Autodesk Inventor part; units mm, degrees
sketch "Sketch19" plane through (0, 0, 0) normal (0, 0, 1) x (1, 0, 0)
  circle A0 centre (0, 0) radius 12.5
  dimension "d130" = 25
extrude "Extrusion17" add sketch "Sketch19" along normal blind 40
sketch "Sketch20" plane through (0, 0, 40) normal (0, 0, 1) x (1, 0, 0)
  circle A0 centre (0, 0) radius 10
  dimension "d133" = 20
fillet "Fillet6" radius 10 1 edges at (-12.5, 0, 0)
extrude "Extrusion18" cut sketch "Sketch20" against normal blind 25
ref_plane "Work Plane3" through (10, 0, 0) normal (1, 0, 0) x (0, 1, 0)
sketch "Sketch21" plane through (10, 0, 0) normal (1, 0, 0) x (0, 1, 0)
  line L0 (0, 0) -> (0, 20)
  circle A0 centre (0, 20) radius 5
  dimension "d138" = 20
  dimension "d139" = 10
extrude "Extrusion19" add sketch "Sketch21" along normal blind 10
mirror "Mirror1" about plane through (0, 0, 0) normal (1, 0, 0) of "Extrusion19"
sketch "Sketch22" plane through (-20, 0, 20) normal (-1, 0, 0) x (0, 0, 1)
  circle A0 centre (0, 0) radius 2.5
  point P0 (-20, 0)
  dimension "d142" = 5
extrude "Extrusion20" cut sketch "Sketch22" against normal blind 3
sketch "Sketch26" plane through (0, 0, 0) normal (1, 0, 0) x (0, 1, 0)
  line L0 (-10, 40) -> (10, 40)
  line L1 (12.5, 40) -> (-12.5, 40)
  line L2 (10, 40) -> (12.5, 40)
  line L3 (17.5, 60) -> (12.5, 40)
  line L4 (17.5, 60) -> (17.5, 62.5)
  line L5 (17.5, 62.5) -> (15, 62.5)
  line L6 (15, 62.5) -> (15, 60)
  line L7 (10, 40) -> (15, 60)
  line L8 (0, -10.5) -> (0, 63)
  point P0 (0, 0)
  dimension "d147" = 2.5
  dimension "d148" = 2.5
revolve "Revolution1" add sketch "Sketch26" angle 360 about axis through (0, 0, -10) along (0, 0, 1)
sketch "Sketch27" plane through (0, 0, 0) normal (1, 0, 0) x (0, 1, 0)
  line L0 (12.5, 40) -> (13.7856, 41.5321)
  line L1 (12.5, 40) -> (14.5, 40) construction
  line L2 (13.7856, 41.5321) -> (17.5, 60)
  line L3 (12.5, 40) -> (-12.5, 40)
  line L4 (12.5, 40) -> (11.5, 40)
  line L5 (-17.5, 60) -> (17.5, 60)
  line L6 (17.5, 60) -> (16.5, 60)
  line L7 (16.5, 60) -> (11.5, 40)
  point P0 (0, 0)
  dimension "d150" = 2
  dimension "d151" = 50
  dimension "d152" = 1
  dimension "d153" = 1
extrude "Extrusion21" add sketch "Sketch27" along normal mid plane 2
pattern_circular "Circular Pattern2" count 8 over 360 about axis through (0, 0, -10) along (0, 0, 1) of "Extrusion21"
properties part number "Waterkanon" material "S235"
The listing builds one solid part. Answer for the finished solid, in the listing's coordinates (mm). A direction names the side the tool comes from. Coordinates: 2 decimals unless noted, no trailing zeros. Loops run counter-clockwise (first coordinate to the right, second up) from the corner with the lowest first, then second, coordinate; pieces in that order, holes last. Notation, with made-up numbers: (5.25, 63.5) -> (29.25, 63.5) arc R28 ccw to (29.25, 99.5) -> close; hole circle Ø7 at (8.25, 17). An arc over 180 degrees is marked (long way). Write item = value, one per line. Start each with the question number.
1) A tool of negligible diameter and unlimited length cuts with its end or side. For faces 1 (the face through (-1, -14.8, 47.8)), 2 (the face through (-15.67, -1.08, 15.12)), 3 (the face through (1, -14.8, 47.8)), from which of +Z, -Z, +X, -X, +Y, -Y can it reach the whole face along a straight path? Write none if from no direction.
2) Straight lines are drawn through the part: line 1 (Y direction, x = 0, z = 61.3); line 2 (Y direction, x = 0, z = 26.5). For each, find the intervals that lie inside material, in ascending order. Write a range as from..to.
3) Given pin 1 Ø12 at (y, z) = (9, 40.5) entering from -X; pin 2 Ø10 at (x, z) = (-4, 28) entering from -Y; pin 3 Ø1.5 at (y, z) = (7.5, 13.5) entering from +X, each flat-ended and moving along its own axis, determine where each tip first touches the part or whether it passes through.
4) A cutting plane is placed at A-A (z = 20). Give the vertices of the cut face in (x, y).
5) The mould has two halves that part along Y. Classify faces 4 (the face through (0.66, -14.985, 61.232)), 5 (the face through (15.67, -1.08, 24.88)), 6 (the face through (-13.134, -0.014, 40.755)), 7 (the face through (-18.5, 0.1, 17.5)): released by +Y, released by -Y, zero draft, split by the parting line, or undercut.
6) A cutting plane is placed at C-C (z = 34.5). Give the vertices of the cut face in (x, y).
Responses:
q1.face_1 = -Z, -X, -Y
q1.face_2 = -X
q1.face_3 = -Z, +X, -Y
q2.line_1 = -17.5..-15, 15..17.5
q2.line_2 = -12.5..-10, 10..12.5
q3.pin_1 = -12.86
q3.pin_2 = -12.5
q3.pin_3 = 10.52
q4.outline = (-20, -5) -> (-11.46, -5) arc R12.5 ccw to (11.46, -5) -> (20, -5) -> (20, 5) -> (11.46, 5) arc R12.5 ccw to (-11.46, 5) -> (-20, 5) -> (-20, 2.5) -> (-17, 2.5) -> (-17, -2.5) -> (-20, -2.5) -> close; hole circle Ø20 at (0, 0)
q5.face_4 = undercut
q5.face_5 = split by the parting line
q5.face_6 = zero draft
q5.face_7 = undercut
q6.outline = circle Ø25 at (0, 0); hole circle Ø20 at (0, 0)
